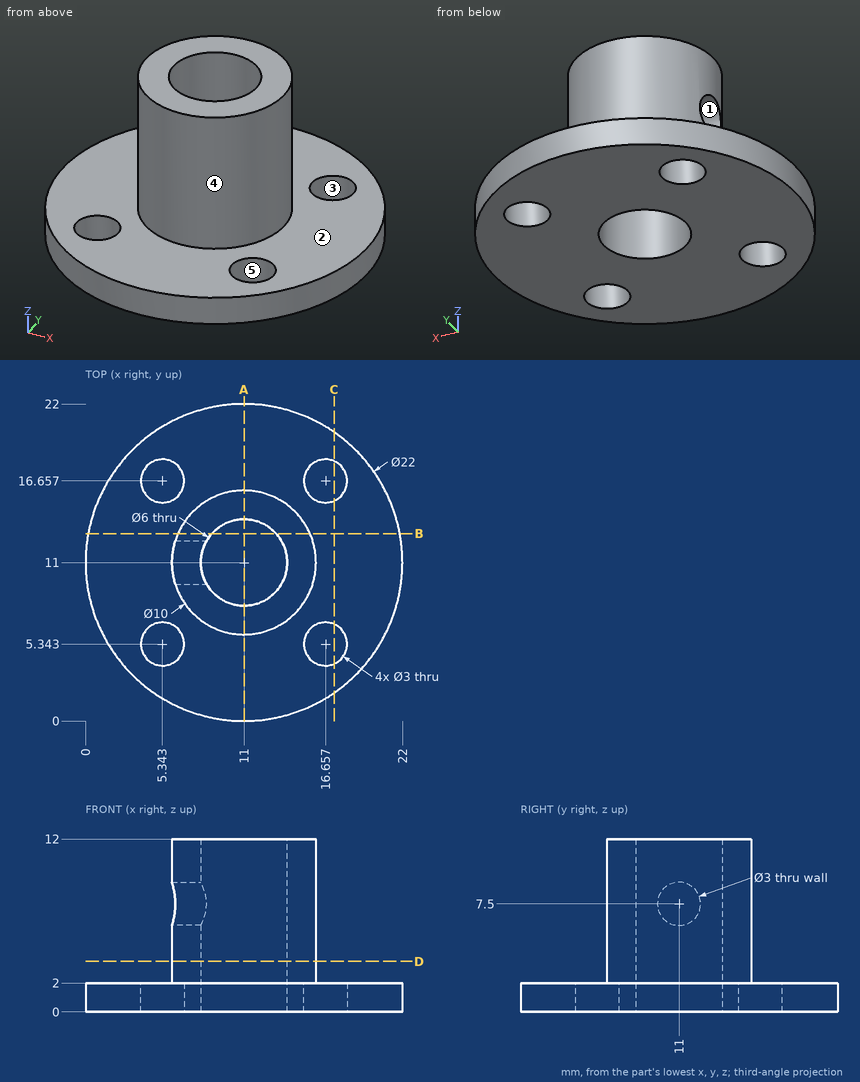
Can you work these out from the drawing? Everything is in mm from the part's minimum corner. A direction names the side the tool comes from. Give positions to 0.01 mm unless a question says otherwise; leave off trailing zeros. Order: outer loops, then holes, each group sorted by start corner. A loop starts at its lowest first (then second) coordinate and runs counter-clockwise, first axis right, second up. Notation, with made-up numbers: M 83.5,-24 L 111.5,-24 A22 ccw 111.5,13 Z; hole C 52,-38.5 d1. An arc over 180 degrees is marked long. Write item = value, one per line. Start each with the question number.
Q1. We'd pull the mould along Z, two halves only. Please class the marked faces 1, 2 and 3: pulls with the +Z half, pulls with the -Z half, needs draft (parallel to the pull), parting line crosses it, or undercut.
Q2. Suppose I cut it at C-C (x = 17.25). Write out the boundary of the cut face in (y, z), plus the area to 3 significant figures.
Q3. Suppose I cut it at D-D (z = 3.5). Write out the boundary of the cut face in (x, y).
Q4. Suppose I cut it at A-A (x = 11). Write out the boundary of the cut face in (y, z).
Q5. Suppose I cut it at B-B (y = 13). Write out the boundary of the cut face in (x, z).
Q6. I need wall thicknesses on probe 1 along Y at (x, z) = (16.25, 0.75); probe 2 along Z at (x, y) = (7, 19); probe 3 along Y at (x, z) = (11, 6.75). Which ranges of each line are inside material? Lowest first, please. Write a range as [from, to].
Q7. For the marked faces 4 and 5, which set-ups out of +Z, -Z, +X, -X, +Y, -Y let a thin tool reach every point of the face, with its end or its side?
Q8. Will these pins go through, and if not, where does the flat tip stop? pin 1 Ø3 at (y, z) = (19, 10) entering from +X; pin 2 Ø8 at (x, y) = (11, 11) entering from +Z; pin 3 Ø5 at (x, y) = (5.34, 5.34) entering from +Z; pin 4 Ø4 at (y, z) = (11, 7.5) entering from -X.
Check result:
q1.face_1 = undercut
q1.face_2 = pulls with the +Z half
q1.face_3 = needs draft
q2.outline = M 1.95,0 L 3.97,0 L 3.97,2 L 1.95,2 Z; M 6.72,0 L 15.28,0 L 15.28,2 L 6.72,2 Z; M 18.03,0 L 20.05,0 L 20.05,2 L 18.03,2 Z
q2.area = 25.2 mm2
q3.outline = C 11,11 d10; hole C 11,11 d6
q4.outline = M 0,0 L 8,0 L 8,12 L 6,12 L 6,2 L 0,2 Z; M 14,0 L 22,0 L 22,2 L 16,2 L 16,12 L 14,12 Z
q5.outline = M 0.18,0 L 8.76,0 L 8.76,12 L 6.42,12 L 6.42,2 L 0.18,2 Z; M 13.24,0 L 21.82,0 L 21.82,2 L 15.58,2 L 15.58,12 L 13.24,12 Z
q6.probe_1 = [1.33, 3.9], [6.79, 15.21], [18.1, 20.67]
q6.probe_2 = [0, 2]
q6.probe_3 = [6, 8], [14, 16]
q7.face_4 = +Z
q7.face_5 = +Z, -Z
q8.pin_1 = through
q8.pin_2 = 12
q8.pin_3 = 2
q8.pin_4 = 6
